Check sheet for the modelled part. Datum: model origin and axes. Units: mm. Face numbers are marked on the shaded views. A direction names the side the tool comes from. Coordinates: 2 decimals unless noted, no trailing zeros. Loops run counter-clockwise (first coordinate to the right, second up) from the corner with the lowest first, then second, coordinate; pieces in that order, holes last. Notation, with made-up numbers: (-32.75, 14) - (-18.75, 14) arc R18 ccw to (-18.75, 39) - close; hole circle Ø7 at (-25.75, 73). An arc over 180 degrees is marked (long way). Use a Markdown table: item, result. Add a question column.
1) Sectioned sample at A-A, the plane x = -72. Enter the section's corners in (y, z), then the cut area to 3 significant figures.
2) Sectioned sample at C-C, the plane z = 21.5. Enter the section's corners in (x, y) (1 decimal), then the cut area to 3 significant figures.
3) Go/stop test with flat-tipped pins: P1, Ø1.5, axis at x = -67, z = 51, coming from the -Y side; P2, Ø4, axis at x = -71, z = 17.5, coming from the -Y side; P3, Ø9.5, axis at x = -72, y = -91.79, coming from the +Z side. Record where each tip stops, or that it passes through.
4) Sectioned sample at B-B, the plane x = -87. Enter the section's corners in (y, z).
5) Thickness scan on line 1 (X direction, y = -41.5, z = 21); line 2 (Y direction, x = -72, z = 4); line 3 (Y direction, x = -72, z = 16.5). Record the ranges inside material, lowest first.
6) Sectioned sample at D-D, the plane z = 9.5. Enter the section's corners in (x, y) (1 decimal), then the cut area to 3 significant figures.
7) Tool access check on the marked faces 1 and 2. Record the directions out of +Z, -Z, +X, -X, +Y, -Y that give a thin tool (end or side, any length) a straight path to the whole face; none if there is none.
from build123d import *

# Parameters (mm, degrees)
SKETCH1_W           = 12.7
SKETCH1_H           = 319.323239592
BOSS_EXTRUDE1_DEPTH = 112.776
SKETCH2_R           = 4
CUT_EXTRUDE1_DEPTH  = 13.7
SKETCH3_R           = 4.1275
CUT_EXTRUDE2_DEPTH  = 25.4
SKETCH4_R           = 4
BOSS_EXTRUDE2_DEPTH = 18.5
CUT_EXTRUDE3_DEPTH  = 12.5
FILLET1_R           = 6


with BuildPart() as part:
    # Sketch1 → Boss-Extrude1 (new body)
    with BuildSketch(Plane.XY):
        with Locations((-72.058445247, -162.550776628)):
            Rectangle(SKETCH1_W, SKETCH1_H)
    extrude(amount=BOSS_EXTRUDE1_DEPTH)

    # Sketch2 → Cut-Extrude1 (cut, through all)
    with BuildSketch(Plane(origin=(-65.708445247, 0, 0), x_dir=(0, 0, -1), z_dir=(1, 0, 0))):
        with BuildLine():
            Line((0, -322.212396424), (0, -102))
            Line((0, -102), (-83.459642539, -217.229583096))
            ThreePointArc((-83.459642539, -217.229583096), (-98.52075591, -220.444553487), (-103.27456158, -205.796191727))
            Line((-103.27456158, -205.796191727), (-12.7, -2.889156832))
            Line((-12.7, -2.889156832), (-112.776, -2.889156832))
            Line((-112.776, -2.889156832), (-112.776, -322.212396424))
            Line((-112.776, -322.212396424), (0, -322.212396424))
        make_face()
        with Locations((-92.773303784, -210.483790762)):
            Circle(SKETCH2_R)
    extrude(amount=-CUT_EXTRUDE1_DEPTH, mode=Mode.SUBTRACT)

    # Sketch3 → Cut-Extrude2 (cut)
    with BuildSketch(Plane(origin=(0, 0, 0), x_dir=(-1, 0, 0), z_dir=(0, 0, -1))):
        with Locations((72, -12.414156832)):
            Circle(SKETCH3_R)
        with Locations((72, -91.789156832)):
            Circle(SKETCH3_R)
    extrude(amount=-CUT_EXTRUDE2_DEPTH, mode=Mode.SUBTRACT)

    # Sketch4 → Boss-Extrude2 (add, symmetric)
    with BuildSketch(Plane(origin=(-72.058445247, 0, 0), x_dir=(0, 0, -1), z_dir=(1, 0, 0))):
        with BuildLine():
            Line((-67.779388484, -195.580447266), (-92.378474043, -181.386547612))
            Line((-92.378474043, -181.386547612), (-103.27456158, -205.796191727))
            ThreePointArc((-103.27456158, -205.796191727), (-98.52075591, -220.444553487), (-83.459642539, -217.229583096))
            Line((-83.459642539, -217.229583096), (-67.779388484, -195.580447266))
        make_face()
        with Locations((-92.773303784, -210.483790762)):
            Circle(SKETCH4_R, mode=Mode.SUBTRACT)
    extrude(amount=BOSS_EXTRUDE2_DEPTH, both=True)

    # Sketch6 → Cut-Extrude3 (cut, symmetric)
    with BuildSketch(Plane(origin=(-72.058445247, 0, 0), x_dir=(0, 0, -1), z_dir=(1, 0, 0))):
        Polygon((-102.882650108, -190.796243791), (-56.569606998, -217.519297579), (-85.086213735, -269.679128088), (-153.833763242, -230.32789021), align=None)
    extrude(amount=CUT_EXTRUDE3_DEPTH, both=True, mode=Mode.SUBTRACT)

    # Fillet1
    fillet1_edges = [part.edges().sort_by_distance(p)[0] for p in [
        (-65.708445247, -188.483497439, 80.078931263),
        (-78.408445247, -188.483497439, 80.078931263),
        (-90.558445247, -188.483497439, 80.078931263),
        (-53.558445247, -188.483497439, 80.078931263),
    ]]
    fillet(fillet1_edges, radius=FILLET1_R)


solid = part.part
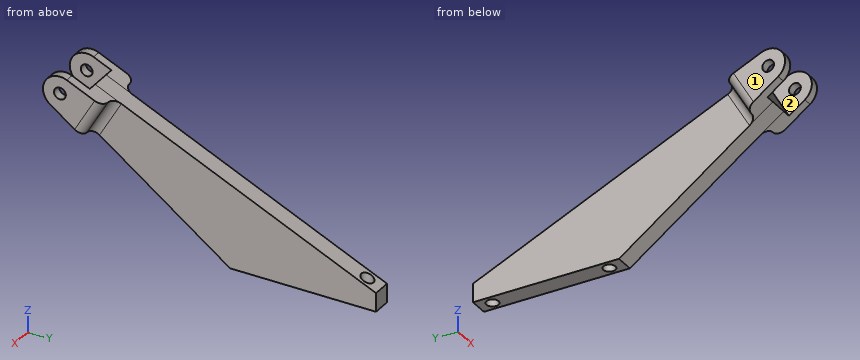
Solved:
| question | item | result |
|---|---|---|
| 1 | outline | (-206.49, 75.68) - (-102, 0) - (-95.92, 0) - (-95.92, 25.4) - (-87.66, 25.4) - (-87.66, 0) - (-16.54, 0) - (-16.54, 18.79) - (-193.69, 97.87) - close; (-8.29, 0) - (-2.89, 0) - (-2.89, 12.7) - (-8.29, 15.11) - close |
| 1 | area | 7,360 mm2 |
| 2 | outline | (-78.4, -131.7) - (-65.7, -131.7) - (-65.7, -22.6) - (-78.4, -22.6) - close; hole circle Ø8.3 at (-72, -91.8) |
| 2 | area | 1,330 mm2 |
| 3 | P1 | stops at y = -173.45 |
| 3 | P2 | stops at y = -128.92 |
| 3 | P3 | stops at z = 54.5 |
| 4 | outline | (-217.23, 83.46) - (-196, 68.09) - (-181.86, 92.59) - (-205.8, 103.27) arc R11.5 ccw to start; hole circle Ø8 at (-210.48, 92.77) |
| 5 | line 1 | x = -78.41 to -65.71 |
| 5 | line 2 | y = -107.52 to -95.92, -87.66 to -16.54, -8.29 to -2.89 |
| 5 | line 3 | y = -124.78 to -95.92, -87.66 to -16.54 |
| 6 | outline | (-78.4, -115.1) - (-65.7, -115.1) - (-65.7, -2.9) - (-78.4, -2.9) - close; hole circle Ø8.3 at (-72, -91.8); hole circle Ø8.3 at (-72, -12.4) |
| 6 | area | 1,320 mm2 |
| 7 | face 1 | +Z, -Z, -X, +Y, -Y |
| 7 | face 2 | +Z, -Y |
